Could you check a few things on this model? Use its own coordinates, in mm. A direction names the side the tool comes from. Round coordinates to 2 decimals unless told otherwise and drop trailing zeros. Loops run counter-clockwise (first coordinate to the right, second up) from the corner with the lowest first, then second, coordinate; pieces in that order, holes last. Notation, with made-up numbers: (12.5, 62.25) -> (40.5, 62.25) arc R23 ccw to (40.5, 79.25) -> close; hole circle Ø9 at (65.5, 2.5). An arc over 180 degrees is marked (long way). Put each result on its own line as item: value. Start each with the question number.
1. I'm going to push flat-ended pins straight in: P1, Ø10.5, axis at y = 16, z = 1.5, coming from the +X side; P2, Ø1.5, axis at y = -8.5, z = 0.5, coming from the +X side; P3, Ø2, axis at x = 70.5, z = 0.5, coming from the +Y side. Where does each tip first touch, or does it pass through?
2. I need wall thicknesses on line 1 (Y direction, x = 60.9, z = 0); line 2 (X direction, y = 10, z = -3.25); line 3 (Z direction, x = 58, y = -8). Which ranges of each line are inside material? Lowest first, please. Write a range as [from, to].
3. Imagine slicing it at A-A, the plane z = 0. Please give me the cut outline in (x, y).
4. If we mould it in two halves opening along Z, with no side actions, what happens to faces 4 (the flat face through (13, 15, -6)), 5 (the flat face through (13, 15, 6)), 6 (the flat face through (57.5, 9, 0)), 7 (the cylindrical face through (60.035, -10.014, 0.325))? For each: pulls with the +Z half, pulls with the -Z half, needs draft (parallel to the pull), parting line crosses it, or undercut.
5. Imagine slicing it at B-B, the plane y = 0. Please give me the cut outline in (x, z).
6. Imagine slicing it at D-D, the plane x = 11. Please give me the cut outline in (y, z).
7. Which directions (+Z, -Z, +X, -X, +Y, -Y) give clear straight access to the entire face, cutting with the end or side of a thin tool? Please do faces 1 (the flat face through (70, 1.5, 0)), 2 (the flat face through (65, 2, 0)), 3 (the flat face through (13, 20, 0)).
8. Imagine slicing it at C-C, the plane x = 61.5. Please give me the cut outline in (y, z).
```python
from build123d import *

# Parameters (mm, degrees)
SKETCH1_R           = 12.2
BOSS_EXTRUDE1_DEPTH = 62.5
SKETCH2_R           = 3.5
BOSS_EXTRUDE2_DEPTH = 2.5
BOSS_EXTRUDE3_DEPTH = 10
SKETCH4_R           = 1.5
CUT_EXTRUDE1_DEPTH  = 5
SKETCH5_W           = 3
SKETCH5_H           = 12
BOSS_EXTRUDE4_DEPTH = 20


with BuildPart() as part:
    # Sketch1 → Boss-Extrude1 (new body)
    with BuildSketch(Plane(origin=(0, 0, 0), x_dir=(0, 0, -1), z_dir=(1, 0, 0))):
        Circle(SKETCH1_R)
    extrude(amount=BOSS_EXTRUDE1_DEPTH)

    # Sketch2 → Boss-Extrude2 (add)
    with BuildSketch(Plane(origin=(62.5, 0, 0), x_dir=(0, 0, -1), z_dir=(1, 0, 0))):
        Circle(SKETCH2_R)
    extrude(amount=BOSS_EXTRUDE2_DEPTH)

    # Sketch3 → Boss-Extrude3 (add)
    with BuildSketch(Plane(origin=(65, 0, 0), x_dir=(0, 0, -1), z_dir=(1, 0, 0))):
        with BuildLine():
            Line((-1.322875656, 1.5), (1.322875656, 1.5))
            ThreePointArc((1.322875656, 1.5), (0, -2), (-1.322875656, 1.5))
        make_face()
    extrude(amount=BOSS_EXTRUDE3_DEPTH)

    # Sketch4 → Cut-Extrude1 (cut)
    with BuildSketch(Plane(origin=(62.5, 0, 0), x_dir=(0, 0, -1), z_dir=(1, 0, 0))):
        with Locations((0, 8.55)):
            Circle(SKETCH4_R)
        with Locations((0, -8.55)):
            Circle(SKETCH4_R)
    extrude(amount=-CUT_EXTRUDE1_DEPTH, mode=Mode.SUBTRACT)

    # Sketch5 → Boss-Extrude4 (add)
    with BuildSketch(Plane(origin=(0, 0, 0), x_dir=(1, 0, 0), z_dir=(0, 1, 0))):
        with Locations((13.2, 0)):
            Rectangle(SKETCH5_W, SKETCH5_H)
    extrude(amount=BOSS_EXTRUDE4_DEPTH)


solid = part.part
```
Entries:
1. P1: x = 62.5
1. P2: x = 57.5
1. P3: y = 1.5
2. line 1: [-12.2, -10.05], [-7.05, 7.05], [10.05, 12.2]
2. line 2: [0, 62.5]
2. line 3: [-9.21, -1.4], [1.4, 9.21]
3. outline: (0, -12.2) -> (62.5, -12.2) -> (62.5, -10.05) -> (57.5, -10.05) -> (57.5, -7.05) -> (62.5, -7.05) -> (62.5, -3.5) -> (65, -3.5) -> (65, -2) -> (75, -2) -> (75, 1.5) -> (65, 1.5) -> (65, 3.5) -> (62.5, 3.5) -> (62.5, 7.05) -> (57.5, 7.05) -> (57.5, 10.05) -> (62.5, 10.05) -> (62.5, 12.2) -> (14.7, 12.2) -> (14.7, 20) -> (11.7, 20) -> (11.7, 12.2) -> (0, 12.2) -> close
4. face 4: pulls with the -Z half
4. face 5: pulls with the +Z half
4. face 6: undercut
4. face 7: undercut
5. outline: (0, -12.2) -> (62.5, -12.2) -> (62.5, -3.5) -> (65, -3.5) -> (65, -2) -> (75, -2) -> (75, 2) -> (65, 2) -> (65, 3.5) -> (62.5, 3.5) -> (62.5, 12.2) -> (0, 12.2) -> close
6. outline: circle Ø24.4 at (0, 0)
7. face 1: +Z, -Z, +X, +Y
7. face 2: +X
7. face 3: +Z, -Z, +X, -X, +Y
8. outline: circle Ø24.4 at (0, 0); hole circle Ø3 at (-8.55, 0); hole circle Ø3 at (8.55, 0)
